The listing builds one solid part. Answer for the finished solid, in the listing's coordinates (mm). A direction names the side the tool comes from. Give positions to 0.01 mm unless a question says otherwise; leave off trailing zeros. Write each loop counter-clockwise with the first axis right and the second up, starting at its lowest first coordinate (ties: lowest second). Pieces come first, ordered by that corner, then holes. Notation, with made-up numbers: M -2,88.5 L 4,88.5 A14 cw 4,113.5 Z; hole C -36,76 d6. An arc over 180 degrees is marked long. Return JSON: item names as keys, results as strings.
from build123d import *

# Parameters (mm, degrees)
SKETCH1_W           = 8
SKETCH1_H           = 46
SKETCH1_R           = 2.1
SKETCH1_H_2         = 106
BOSS_EXTRUDE1_DEPTH = 8
SKETCH2_R           = 1.65
CUT_EXTRUDE1_DEPTH  = 5
SKETCH3_R           = 1.65
CUT_EXTRUDE2_DEPTH  = 10
SKETCH4_R           = 1.65
CUT_EXTRUDE3_DEPTH  = 10
SKETCH5_R           = 1.65
CUT_EXTRUDE4_DEPTH  = 10


with BuildPart() as part:
    # Sketch1 → Boss-Extrude1 (new body)
    with BuildSketch(Plane(origin=(0, 0, 0), x_dir=(0, 0, -1), z_dir=(1, 0, 0))):
        with Locations((-86, -30)):
            Rectangle(SKETCH1_W, SKETCH1_H)
        with Locations((-86, -41.5)):
            Circle(SKETCH1_R, mode=Mode.SUBTRACT)
        with Locations((-86, -18.5)):
            Circle(SKETCH1_R, mode=Mode.SUBTRACT)
        Polygon((82, 53), (9.5, 53), (9.5, -7), (-82, -7), (-82, -53), (82, -53), align=None)
        with Locations((86, 0)):
            Rectangle(SKETCH1_W, SKETCH1_H_2)
        with Locations((86, -39.75)):
            Circle(SKETCH1_R, mode=Mode.SUBTRACT)
        with Locations((86, -13.25)):
            Circle(SKETCH1_R, mode=Mode.SUBTRACT)
        with Locations((86, 13.25)):
            Circle(SKETCH1_R, mode=Mode.SUBTRACT)
        with Locations((86, 39.75)):
            Circle(SKETCH1_R, mode=Mode.SUBTRACT)
    extrude(amount=-BOSS_EXTRUDE1_DEPTH)

    # Sketch2 → Cut-Extrude1 (cut)
    with BuildSketch(Plane.XZ.offset(53)):
        with Locations((-4, -86)):
            Circle(SKETCH2_R)
        with Locations((-4, -4.5)):
            Circle(SKETCH2_R)
        with Locations((-4, -45.25)):
            Circle(SKETCH2_R)
    extrude(amount=-CUT_EXTRUDE1_DEPTH, mode=Mode.SUBTRACT)

    # Sketch3 → Cut-Extrude2 (cut)
    with BuildSketch(Plane(origin=(0, 53, 0), x_dir=(1, 0, 0), z_dir=(0, 1, 0))):
        with Locations((-4, 49.75)):
            Circle(SKETCH3_R)
        with Locations((-4, 74.75)):
            Circle(SKETCH3_R)
        with Locations((-4, 24.75)):
            Circle(SKETCH3_R)
    extrude(amount=-CUT_EXTRUDE2_DEPTH, mode=Mode.SUBTRACT)

    # Sketch4 → Cut-Extrude3 (cut)
    with BuildSketch(Plane(origin=(0, -7, 0), x_dir=(1, 0, 0), z_dir=(0, 1, 0))):
        with Locations((-4, -2.9375)):
            Circle(SKETCH4_R)
        with Locations((-4, -27.8125)):
            Circle(SKETCH4_R)
        with Locations((-4, -52.6875)):
            Circle(SKETCH4_R)
        with Locations((-4, -77.5625)):
            Circle(SKETCH4_R)
    extrude(amount=-CUT_EXTRUDE3_DEPTH, mode=Mode.SUBTRACT)

    # Sketch5 → Cut-Extrude4 (cut)
    with BuildSketch(Plane.XY.offset(-9.5)):
        with Locations((-4, 11)):
            Circle(SKETCH5_R)
        with Locations((-4, 43)):
            Circle(SKETCH5_R)
        with Locations((-4, 27)):
            Circle(SKETCH5_R)
    extrude(amount=-CUT_EXTRUDE4_DEPTH, mode=Mode.SUBTRACT)


solid = part.part
Item 1: Given pin 1 Ø5 at (y, z) = (13.25, -86) entering from +X; pin 2 Ø12 at (y, z) = (27, -2) entering from +X; pin 3 Ø2 at (x, z) = (-4, 27.81) entering from +Y; pin 4 Ø2 at (x, z) = (-4, -74.75) entering from +Y, each flat-ended and moving along its own axis, determine where each tip first touches the part or whether it passes through.
Geometry results:
{"pin 1": "stops at x = 0", "pin 2": "passes through", "pin 3": "stops at y = -17", "pin 4": "stops at y = 43"}
Item 2: A cutting plane is placed at C-C, the plane x = -4.25. Count the separate pieces of the cut face and the enclosed holes in it, plus the area to 3 significant figures.
Geometry results:
{"separate pieces": "1", "enclosed holes": "6", "area": "12,700 mm2"}
Item 3: Determine the mould class of faces 1 (the cylindrical face through (-4.215, 28.636, -14.43)), 2 (the flat face through (-4, -17, 53)), 3 (the flat face through (-4, -30, 90)) for opening direction Y: +Y half, -Y half, draft (parallel to the pull), parting line (faces both ways), or undercut.
Geometry results:
{"face 1": "undercut", "face 2": "+Y half", "face 3": "draft"}
Item 4: Which of the six approach directions +Z, -Z, +X, -X, +Y, -Y give full straight-line access (tool end or side, diameter ignored) to faces 4 (the flat face through (-4, 11, -19.5)), 5 (the flat face through (-4, -48, -86)), 6 (the cylindrical face through (-5.216, -11.93, 51.572))?
Geometry results:
{"face 4": "+Z", "face 5": "-Y", "face 6": "+Y"}
Item 5: Find the intervals of material crossed by line 1 (Y direction, x = -4, z = -13.5); line 2 (Z direction, x = -4, y = 46.5); line 3 (Y direction, x = -4, z = -86), in increasing order.
Geometry results:
{"line 1": "y = -53 to 9.35, 12.65 to 25.35, 28.65 to 41.35, 44.65 to 53", "line 2": "z = -90 to -76.4, -73.1 to -51.4, -48.1 to -26.4, -23.1 to -9.5", "line 3": "y = -48 to -41.85, -37.65 to -15.35, -11.15 to 11.15, 15.35 to 37.65, 41.85 to 53"}
Item 6: A cutting plane is placed at A-A, the plane z = 33.5. Write down the section's boundary in (x, y).
Geometry results:
{"outline": "M -8,-53 L 0,-53 L 0,-7 L -8,-7 Z"}
Item 7: A cutting plane is placed at B-B, the plane y = 23.5. Write down the section's boundary in (x, z).
Geometry results:
{"outline": "M -8,-90 L 0,-90 L 0,-9.5 L -8,-9.5 Z"}
